```python
from build123d import *

# Parameters (mm, degrees)
SKETCH2_R           = 2.38125
SKETCH2_R_2         = 1.85
BOSS_EXTRUDE1_DEPTH = 4.318


with BuildPart() as part:
    # Sketch2 → Boss-Extrude1 (new body)
    with BuildSketch(Plane(origin=(0, 0, 0), x_dir=(0, 0, -1), z_dir=(1, 0, 0))):
        with BuildLine():
            Line((290.863193916, 48.3172966), (257.759258716, 32))
            Line((257.759258716, 32), (257.759258716, 5))
            ThreePointArc((257.759258716, 5), (256.294792622, 1.464466094), (252.759258716, 0))
            Line((252.759258716, 0), (231.380747369, 0))
            ThreePointArc((231.380747369, 0), (175.759258716, 37.5), (120.137770063, 0))
            Line((120.137770063, 0), (-40.619252631, 0))
            ThreePointArc((-40.619252631, 0), (-78.000395352, 34.660211514), (-128.548433592, 28.059005308))
            ThreePointArc((-128.548433592, 28.059005308), (-133.642663591, 27.886965654), (-136.240741284, 32.272255751))
            Line((-136.240741284, 32.272255751), (-136.240741284, 82.154119676))
            ThreePointArc((-136.240741284, 82.154119676), (-111.765249408, 180.544448903), (-44.044009042, 256))
            Line((-44.044009042, 256), (215.955990958, 256))
            ThreePointArc((215.955990958, 256), (271.683097829, 163.39777941), (296.50139881, 58.208741794))
            ThreePointArc((296.50139881, 58.208741794), (295.198004633, 52.399053051), (290.863193916, 48.3172966))
        make_face()
        with Locations((286.371258716, 57.430370624)):
            Circle(SKETCH2_R, mode=Mode.SUBTRACT)
        with Locations((-10.544009042, 238)):
            Circle(SKETCH2_R_2, mode=Mode.SUBTRACT)
        with Locations((-26.544009042, 238)):
            Circle(SKETCH2_R_2, mode=Mode.SUBTRACT)
        with Locations((-18.544009042, 246)):
            Circle(SKETCH2_R_2, mode=Mode.SUBTRACT)
        with Locations((199.955990958, 232)):
            Circle(SKETCH2_R_2, mode=Mode.SUBTRACT)
        with Locations((199.955990958, 248)):
            Circle(SKETCH2_R_2, mode=Mode.SUBTRACT)
        with Locations((207.955990958, 176)):
            Circle(SKETCH2_R_2, mode=Mode.SUBTRACT)
        with Locations((191.955990958, 80)):
            Circle(SKETCH2_R_2, mode=Mode.SUBTRACT)
        with Locations((199.955990958, 40)):
            Circle(SKETCH2_R_2, mode=Mode.SUBTRACT)
        with Locations((199.955990958, 56)):
            Circle(SKETCH2_R_2, mode=Mode.SUBTRACT)
        with Locations((207.955990958, 48)):
            Circle(SKETCH2_R_2, mode=Mode.SUBTRACT)
        with Locations((191.955990958, 48)):
            Circle(SKETCH2_R_2, mode=Mode.SUBTRACT)
        with Locations((231.759258716, 24)):
            Circle(SKETCH2_R_2, mode=Mode.SUBTRACT)
        with Locations((239.759258716, 16)):
            Circle(SKETCH2_R_2, mode=Mode.SUBTRACT)
        with Locations((111.759258716, 16)):
            Circle(SKETCH2_R_2, mode=Mode.SUBTRACT)
        with Locations((-32.240741284, 16)):
            Circle(SKETCH2_R_2, mode=Mode.SUBTRACT)
        with Locations((-24.240741284, 8)):
            Circle(SKETCH2_R_2, mode=Mode.SUBTRACT)
        with Locations((191.955990958, 176)):
            Circle(SKETCH2_R_2, mode=Mode.SUBTRACT)
        with Locations((110.573562062, 75.111023639)):
            Circle(SKETCH2_R_2, mode=Mode.SUBTRACT)
        with Locations((112.732319414, 86.216867448)):
            Circle(SKETCH2_R_2, mode=Mode.SUBTRACT)
        with Locations((101.626475606, 88.3756248)):
            Circle(SKETCH2_R_2, mode=Mode.SUBTRACT)
        with Locations((28.820215612, 169.5)):
            Circle(SKETCH2_R_2, mode=Mode.SUBTRACT)
        with Locations((28.820215612, 185.5)):
            Circle(SKETCH2_R_2, mode=Mode.SUBTRACT)
        with Locations((20.820215612, 177.5)):
            Circle(SKETCH2_R_2, mode=Mode.SUBTRACT)
        with Locations((229.557259723, 141.660587995)):
            Circle(SKETCH2_R, mode=Mode.SUBTRACT)
        Polygon((148.238437649, 51.459798909), (151.818221888, 53.874393866), (158.919971762, 43.345616694), (155.340187523, 40.931021737), align=None, mode=Mode.SUBTRACT)
        Polygon((46.735820142, 108.250358678), (56.681039096, 109.295643311), (57.17465911, 104.599162588), (47.229440157, 103.553877955), align=None, mode=Mode.SUBTRACT)
        Polygon((82.693937784, 112.029709134), (92.639156737, 113.074993767), (93.132776752, 108.378513044), (83.187557798, 107.333228412), align=None, mode=Mode.SUBTRACT)
    extrude(amount=BOSS_EXTRUDE1_DEPTH)


solid = part.part
```
Geometry: final body of the model. Coordinates: model frame, mm. Coordinates: 2 decimals unless noted, no trailing zeros. Order: outer loops, then holes, each group sorted by start corner. A loop starts at its lowest first (then second) coordinate and runs counter-clockwise, first axis right, second up. Notation, with made-up numbers: (84.25, 23) -> (96.25, 23) arc R23 ccw to (96.25, 31) -> close; hole circle Ø1 at (63.5, -29). An arc over 180 degrees is marked (long way). Use CSV: the item, a comma, the result in double quotes.
1) Section B-B on z = -129. Output: boundary loops of the cut face in (x, y), then the cut area to 3 significant figures.
Findings:
outline,"(0, 15.1) -> (4.32, 15.1) -> (4.32, 256) -> (0, 256) -> close"
area,"1,040 mm^2"
2) Section C-C on z = 91.5. Output: boundary loops of the cut face in (x, y), then the cut area to 3 significant figures.
Findings:
outline,"(0, 37.31) -> (4.32, 37.31) -> (4.32, 211.73) -> (0, 211.73) -> close"
area,"753 mm^2"
3) Pin query (flat end, axial travel): pin 1 Ø3 at (y, z) = (57.43, -286.37) entering from -X; pin 2 Ø1 at (x, y) = (2, 26.5) entering from +Z; pin 3 Ø2 at (x, y) = (1.5, 17) entering from -Z; pin 4 Ø1.5 at (x, y) = (3, 144.5) entering from +Z. Return the tip coordinate at first contact, or that it passes through.
Findings:
pin 1,"passes through"
pin 2,"stops at z = 62.33"
pin 3,"stops at z = -257.76"
pin 4,"stops at z = 127"
4) Section A-A on x = 2.45. State how many separate pieces and enclosed holes the cut face has, then the cut area to 3 significant figures.
Findings:
separate pieces,"1"
enclosed holes,"28"
area,"92,500 mm^2"
5) Line query: line 1 (Y direction, x = 2.8, z = 27); line 2 (Z direction, x = 1.55, y = 46.5); line 3 (Z direction, x = 3.05, y = 176). Output: solid intervals per line, ascending.
Findings:
line 1,"y = 0 to 236.21, 239.79 to 256"
line 2,"z = -287.18 to -209.04, -206.87 to -193.04, -190.87 to -156.79, -151.58 to 136.24"
line 3,"z = -266.26 to -209.81, -206.11 to -193.81, -190.11 to -21.9, -19.74 to 114.1"
